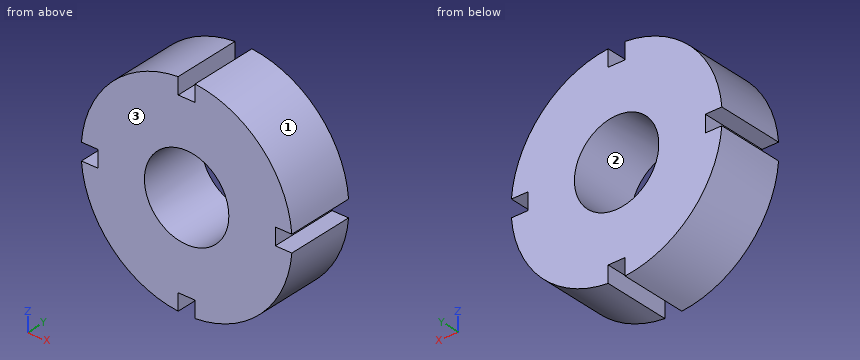
from build123d import *

# Parameters (mm, degrees)
SKETCH_R        = 12.5
SKETCH_R_2      = 5
PAD_DEPTH       = 8
SKETCH001_W     = 8.228719
SKETCH001_H     = 2
SKETCH001_W_2   = 5.633815
POCKET_DEPTH    = 8.001
SKETCH002_W     = 2
SKETCH002_H     = 3.680985
SKETCH002_H_2   = 3.52239
POCKET001_DEPTH = 8.001


with BuildPart() as part:
    # Sketch → Pad (new body)
    with BuildSketch(Plane.XZ):
        Circle(SKETCH_R)
        Circle(SKETCH_R_2, mode=Mode.SUBTRACT)
    extrude(amount=PAD_DEPTH)

    # Sketch001 → Pocket (cut, through all)
    with BuildSketch(Plane.XZ.offset(8)):
        with Locations((14.614359, 0)):
            Rectangle(SKETCH001_W, SKETCH001_H)
        with Locations((-13.316907, 0)):
            Rectangle(SKETCH001_W_2, SKETCH001_H)
    extrude(amount=-POCKET_DEPTH, mode=Mode.SUBTRACT)

    # Sketch002 → Pocket001 (cut, through all)
    with BuildSketch(Plane.XZ.offset(8)):
        with Locations((0, 12.340492)):
            Rectangle(SKETCH002_W, SKETCH002_H)
        with Locations((0, -12.261195)):
            Rectangle(SKETCH002_W, SKETCH002_H_2)
    extrude(amount=-POCKET001_DEPTH, mode=Mode.SUBTRACT)


solid = part.part
Geometry check sheet. Reference: the model listing, model coordinates, mm. Face numbers are marked on the shaded views. Give positions to 0.01 mm unless a question says otherwise; leave off trailing zeros. Order: outer loops, then holes, each group sorted by start corner. A loop starts at its lowest first (then second) coordinate and runs counter-clockwise, first axis right, second up. Notation, with made-up numbers: M 69,-16.75 L 95,-16.75 A20 cw 95,-10.75 Z; hole C 29,1.5 d10. An arc over 180 degrees is marked long. Use a Markdown table: item, result.
Item 1: Depth check by flat-ended pin: P1, Ø1.6, axis at y = -6, z = 11.5, coming from the +X side; P2, Ø1, axis at y = -3, z = 0, coming from the +X side; P3, Ø1, axis at y = -2.5, z = -11.5, coming from the -X side. Enter the tip coordinate at first touch or a pass-through.
Answers follow:
| item | result |
|---|---|
| P1 | stops at x = 6.46 |
| P2 | stops at x = 10.5 |
| P3 | stops at x = -5.94 |
Item 2: Section check A-A (x = 0). Record the cut outline in (y, z), and give its area (3 significant figures).
Answers follow:
| item | result |
|---|---|
| outline | M -8,-10.5 L 0,-10.5 L 0,-5 L -8,-5 Z; M -8,5 L 0,5 L 0,10.5 L -8,10.5 Z |
| area | 88.0 mm2 |
Item 3: Material ranges on line 1 along Z through (x, y) = (0, -6.5); line 2 along Z through (x, y) = (-3.5, -2.25), recorded low to high.
Answers follow:
| item | result |
|---|---|
| line 1 | z = -10.5 to -5, 5 to 10.5 |
| line 2 | z = -12 to -3.57, 3.57 to 12 |
Item 4: Draft check along X on the marked faces 1, 2 and 3. Enter one of: +X half, -X half, draft (parallel to the pull), parting line (faces both ways), or undercut.
Answers follow:
| item | result |
|---|---|
| face 1 | +X half |
| face 2 | undercut |
| face 3 | draft |
Item 5: Section check B-B (z = 0). Record the cut outline in (x, y).
Answers follow:
| item | result |
|---|---|
| outline | M -10.5,-8 L -5,-8 L -5,0 L -10.5,0 Z; M 5,-8 L 10.5,-8 L 10.5,0 L 5,0 Z |
Item 6: Section check C-C (y = -6.5). Record the cut outline in (x, z), and give its area (3 significant figures).
Answers follow:
| item | result |
|---|---|
| outline | M -12.46,-1 A12.5 ccw -1,-12.46 L -1,-10.5 L 1,-10.5 L 1,-12.46 A12.5 ccw 12.46,-1 L 10.5,-1 L 10.5,1 L 12.46,1 A12.5 ccw 1,12.46 L 1,10.5 L -1,10.5 L -1,12.46 A12.5 ccw -12.46,1 L -10.5,1 L -10.5,-1 Z; hole C 0,0 d10 |
| area | 396 mm2 |
Item 7: Section check D-D (z = 8.75). Record the cut outline in (x, y).
Answers follow:
| item | result |
|---|---|
| outline | M -8.93,-8 L 8.93,-8 L 8.93,0 L -8.93,0 Z |
